Geometry check sheet. Reference: the model listing, model coordinates, mm. Round coordinates to 2 decimals unless told otherwise and drop trailing zeros. Order: outer loops, then holes, each group sorted by start corner. A loop starts at its lowest first (then second) coordinate and runs counter-clockwise, first axis right, second up. Notation, with made-up numbers: (-6.75, -33.5) -> (48.25, -33.5) arc R16 ccw to (48.25, -5.5) -> close; hole circle Ø3 at (-29, 60). An arc over 180 degrees is marked (long way). Use a Markdown table: item, result. Add a question column.
Item 1: Sectioned sample at B-B, the plane y = -0.65. Record the cut outline in (x, z) (3 decimals), and give its area (3 significant figures).
Item 2: Gauge pin test, flat ends, axial feed: pin 1 Ø4 at (x, y) = (-4.5, 27.5) entering from +Z; pin 2 Ø1.2 at (y, z) = (-29, 0.5) entering from -X; pin 3 Ø1.2 at (x, z) = (-65, 1) entering from -Y. Record the tip position at first contact, or that the pin passes through.
Item 3: Sectioned sample at D-D, the plane y = -8.5. Record the cut outline in (x, z) (3 decimals), and give its area (3 significant figures).
Item 4: Material ranges on probe 1 along Z at (x, y) = (6.5, -23); probe 2 along X at (y, z) = (-16, 0.75) (3 decimals); probe 3 along Y at (x, z) = (29, 4), recorded low to high. Write a range as [from, to].
Item 5: Sectioned sample at A-A, the plane z = 4.75. Record the cut outline in (x, y) (3 decimals).
Item 6: Sectioned sample at C-C, the plane x = -43.5. Record the cut outline in (y, z).
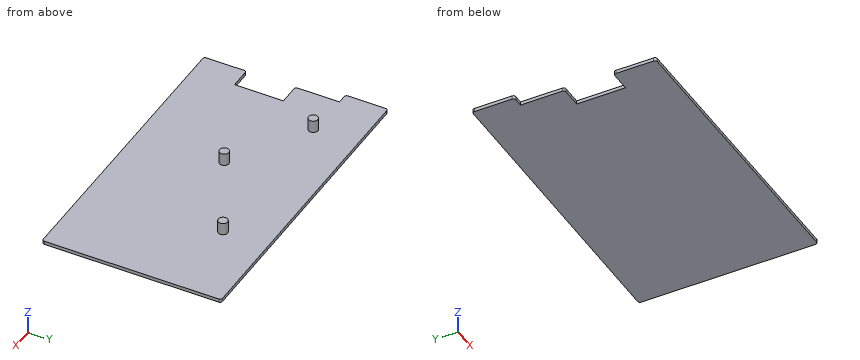
Autodesk Inventor part; units mm, degrees
ref_plane "YZ Plane" through (0, 0, 0) normal (1, 0, 0) x (0, 1, 0)
ref_plane "XZ Plane" through (0, 0, 0) normal (0, 1, 0) x (-1, 0, 0)
ref_plane "XY Plane" through (0, 0, 0) normal (0, 0, 1) x (1, 0, 0)
sketch "Sketch1" plane through (0, 0, 0) normal (0, 0, 1) x (1, 0, 0)
  line L0 (67.175, 38.35) -> (67.175, 15.986)
  arc A0 (67.175, 38.35) -> (66.175, 39.35) centre (66.175, 38.35) ccw
  line L1 (-33.175, 39.35) -> (66.175, 39.35)
  arc A1 (-34.175, 40.35) -> (-33.175, 39.35) centre (-33.175, 40.35) ccw
  line L2 (-34.175, 40.35) -> (-34.175, 43.6)
  line L3 (-34.175, 43.6) -> (-34.5505, 43.6)
  spline S0 degree 3 poles (-35.175, 43.605) (-35.038, 43.605) (-34.8736, 43.6028) (-34.6784, 43.6006) (-34.6086, 43.6) (-34.5505, 43.6) knots 0.473314 0.473314 0.473314 0.473314 0.514423 0.514423 0.531864 0.531864 0.531864 0.531864
  line L4 (-51.175, 43.605) -> (-35.175, 43.605)
  spline S1 degree 3 poles (-51.7995, 43.6) (-51.7414, 43.6) (-51.6716, 43.6006) (-51.4764, 43.6028) (-51.312, 43.605) (-51.175, 43.605) knots 0.531978 0.531978 0.531978 0.531978 0.549419 0.549419 0.590528 0.590528 0.590528 0.590528
  line L5 (-51.7995, 43.6) -> (-52.175, 43.6)
  line L6 (-52.175, 43.6) -> (-52.175, 40.35)
  arc A2 (-53.175, 39.35) -> (-52.175, 40.35) centre (-53.175, 40.35) ccw
  line L7 (-67.175, 39.35) -> (-53.175, 39.35)
  line L8 (-67.175, 20.05) -> (-67.175, 39.35)
  line L9 (-62.412, 20.05) -> (-67.175, 20.05)
  line L10 (-62.412, 1) -> (-62.412, 20.05)
  line L11 (-52.887, 1) -> (-62.412, 1)
  line L12 (-52.887, -20.05) -> (-52.887, 1)
  line L13 (-62.4125, -20.05) -> (-52.887, -20.05)
  line L14 (-62.4125, -39.35) -> (-62.4125, -20.05)
  line L15 (66.175, -39.35) -> (-62.4125, -39.35)
  arc A3 (66.175, -39.35) -> (67.175, -38.35) centre (66.175, -38.35) ccw
  line L16 (67.175, 0.986) -> (67.175, -38.35)
  arc A4 (68.175, 1.986) -> (67.175, 0.986) centre (68.175, 0.986) ccw
  line L17 (68.175, 1.986) -> (71.425, 1.986)
  line L18 (71.425, 1.986) -> (71.425, 2.3615)
  spline S2 degree 3 poles (71.43, 2.986) (71.43, 2.849) (71.4278, 2.6846) (71.4256, 2.4894) (71.425, 2.4196) (71.425, 2.3615) knots 0.473429 0.473429 0.473429 0.473429 0.514537 0.514537 0.531978 0.531978 0.531978 0.531978
  line L19 (71.43, 13.986) -> (71.43, 2.986)
  spline S3 degree 3 poles (71.425, 14.6105) (71.425, 14.5524) (71.4256, 14.4826) (71.4278, 14.2874) (71.43, 14.123) (71.43, 13.986) knots 0.531978 0.531978 0.531978 0.531978 0.549419 0.549419 0.590528 0.590528 0.590528 0.590528
  line L20 (71.425, 14.6105) -> (71.425, 14.986)
  line L21 (71.425, 14.986) -> (68.175, 14.986)
  arc A5 (67.175, 15.986) -> (68.175, 14.986) centre (68.175, 15.986) ccw
  line L22 (-67.175, 39.35) -> (-67.175, 38.35)
  line L23 (-67.175, 39.35) -> (67.175, 39.35)
  line L24 (67.175, 39.35) -> (67.175, -39.35)
  line L25 (67.175, -39.35) -> (-67.175, -39.35)
  line L26 (-67.175, -39.35) -> (-67.175, 39.35)
  line L27 (67.175, -39.35) -> (67.175, -38.35)
  line L28 (67.175, -38.35) -> (-62.4125, -38.35)
  line L29 (67.175, 39.35) -> (67.175, 38.85)
  line L30 (67.175, 38.85) -> (-67.175, 38.35)
  line L31 (67.175, 39.35) -> (66.675, 39.35)
  line L32 (66.675, 39.35) -> (67.175, 39.35)
  line L33 (67.175, 39.35) -> (67.175, -39.35)
  line L34 (67.175, -39.35) -> (66.675, -39.35)
  line L35 (66.675, -39.35) -> (66.675, 39.35)
  point P0 (0, 0)
  point P1 (67.175, -38.35)
  point P2 (67.0413, 38.8495)
  point P3 (66.675, -38.35)
  point P4 (66.675, 38.8481)
  dimension "d0" = 1
  dimension "d1" = 1
  dimension "d2" = 0.5
  dimension "d16" = 0.5
extrude "Extrusion1" add sketch "Sketch1" along normal blind 1.5 contours L35 L28 L14 L13 L12 L11 L10 L9 L8 L30
fillet "Fillet1" radius 1 7 edges at (-67.175, 38.35, 0.75) (-67.175, 20.05, 0.75) (-62.412, 1, 0.75) (-62.4125, -20.05, 0.75) (-62.4125, -38.35, 0.75) (66.675, 38.8481, 0.75) (66.675, -38.35, 0.75)
sketch "Sketch2" plane through (0, 0, 1.5) normal (0, 0, 1) x (1, 0, 0)
  line L0 (65.6713, 38.8444) -> (-66.1787, 38.3537)
  arc A0 (-66.1787, 38.3537) -> (-67.175, 37.3537) centre (-66.175, 37.3537) ccw
  line L1 (-67.175, 37.3537) -> (-67.175, 21.05)
  arc A1 (-67.175, 21.05) -> (-66.175, 20.05) centre (-66.175, 21.05) ccw
  line L2 (-66.175, 20.05) -> (-62.412, 20.05)
  line L3 (-62.412, 20.05) -> (-62.412, 2)
  arc A2 (-62.412, 2) -> (-61.412, 1) centre (-61.412, 2) ccw
  line L4 (-61.412, 1) -> (-52.887, 1)
  line L5 (-52.887, 1) -> (-52.887, -20.05)
  line L6 (-52.887, -20.05) -> (-61.4125, -20.05)
  arc A3 (-61.4125, -20.05) -> (-62.4125, -21.05) centre (-61.4125, -21.05) ccw
  line L7 (-62.4125, -21.05) -> (-62.4125, -37.35)
  arc A4 (-62.4125, -37.35) -> (-61.4125, -38.35) centre (-61.4125, -37.35) ccw
  line L8 (-61.4125, -38.35) -> (65.675, -38.35)
  line L9 (67.175, 38.85) -> (67.175, 19.35)
  line L10 (67.175, 19.35) -> (29.175, 19.35)
  circle A5 centre (29.175, 19.35) radius 2
  line L11 (29.175, 19.35) -> (-42.825, 19.35)
  circle A6 centre (-42.825, 19.35) radius 2
  line L12 (29.175, 19.35) -> (-8.825, 19.35)
  line L13 (-8.825, 19.35) -> (-8.825, -0.65)
  circle A7 centre (-8.825, -0.65) radius 2
  line L14 (66.675, -37.35) -> (66.675, 37.8444)
  arc A8 (65.675, -38.35) -> (66.675, -37.35) centre (65.675, -37.35) ccw
  arc A9 (66.675, 37.8444) -> (65.6713, 38.8444) centre (65.675, 37.8444) ccw
  point P0 (0, 0)
  dimension "d6" = 19.5
  dimension "d7" = 38
  dimension "d8" = 4
  dimension "d9" = 72
  dimension "d10" = 4
  dimension "d11" = 38
  dimension "d12" = 20
  dimension "d13" = 4
extrude "Extrusion2" add sketch "Sketch2" along normal blind 5.35 contours A7 | A6 | A5 L11 L10 | L10 L11 A5
properties part number "BottomInner_right"
Found:
| question | item | result |
|---|---|---|
| 1 | outline | (-52.887, 0) -> (66.675, 0) -> (66.675, 1.5) -> (-6.825, 1.5) -> (-6.825, 6.85) -> (-10.825, 6.85) -> (-10.825, 1.5) -> (-52.887, 1.5) -> close |
| 1 | area | 201 mm2 |
| 2 | pin 1 | stops at z = 1.5 |
| 2 | pin 2 | stops at x = -62.41 |
| 2 | pin 3 | stops at y = 20.05 |
| 3 | outline | (-52.887, 0) -> (66.675, 0) -> (66.675, 1.5) -> (-52.887, 1.5) -> close |
| 3 | area | 179 mm2 |
| 4 | probe 1 | z = [0, 1.5] |
| 4 | probe 2 | x = [-52.887, 66.675] |
| 4 | probe 3 | y = [17.36, 21.34] |
| 5 | outline | circle Ø4 at (-42.825, 19.35); circle Ø4 at (-8.825, -0.65); circle Ø4 at (29.175, 19.35) |
| 6 | outline | (-38.35, 0) -> (38.44, 0) -> (38.44, 1.5) -> (21.23, 1.5) -> (21.23, 6.85) -> (17.47, 6.85) -> (17.47, 1.5) -> (-38.35, 1.5) -> close |
